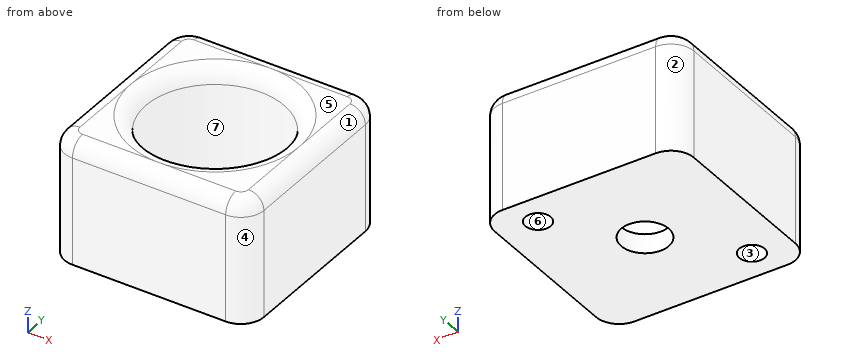
from build123d import *

# Parameters (mm, degrees)
F0_W     = 26
F0_H     = 26
F1_DEPTH = 16
F2_R     = 9
F3_DEPTH = 13.5
F4_R     = 1.65
F4_R_2   = 3.1
F5_DEPTH = 13
F6_R     = 3
F7_R     = 1.99999


# Not quite as in the source:
# - a fillet or chamfer is up to 0.001 mm smaller than in the source, because OpenCascade refuses the exact size


with BuildPart() as f1:
    # F0 (on Top) → F1 (new body)
    with BuildSketch(Plane.XY):
        Rectangle(F0_W, F0_H)
    extrude(amount=F1_DEPTH)

    # F2 (on face) → F3 (cut)
    with BuildSketch(Plane.XY.offset(16)):
        Circle(F2_R)
    extrude(amount=-F3_DEPTH, mode=Mode.SUBTRACT)

    # F4 (on face) → F5 (cut)
    with BuildSketch(Plane(origin=(0, 0, 0), x_dir=(1, 0, 0), z_dir=(0, 0, -1))):
        with Locations((8, -9)):
            Circle(F4_R)
        Circle(F4_R_2)
        with Locations((-8, 9)):
            Circle(F4_R)
    extrude(amount=-F5_DEPTH, mode=Mode.SUBTRACT)

    # F6
    f6_edges = [f1.edges().sort_by_distance(p)[0] for p in [
        (-13, 13, 8),
        (13, 13, 8),
        (-13, -13, 8),
        (13, -13, 8),
    ]]
    fillet(f6_edges, radius=F6_R)

    # F7 (radius 2 in the source; OpenCascade refuses exactly that, so slightly less here)
    f7_edges = [f1.edges().sort_by_distance(p)[0] for p in [
        (-12.12132, -12.12132, 16),
        (-13, 0, 16),
        (-12.12132, 12.12132, 16),
        (0, 13, 16),
        (12.12132, 12.12132, 16),
        (13, 0, 16),
        (12.12132, -12.12132, 16),
        (0, -13, 16),
        (-9, 0, 16),
    ]]
    fillet(f7_edges, radius=F7_R)


solid = f1.part
Here's how the part is built. I have some questions about the finished solid (model axes, mm). Face numbers are marked on the shaded views. A direction names the side the tool comes from. Round coordinates to 2 decimals unless told otherwise and drop trailing zeros. Write each loop counter-clockwise with the first axis right and the second up, starting at its lowest first coordinate (ties: lowest second). Pieces come first, ordered by that corner, then holes.
1. Suppose I cut it at D-D (z = 7.75). List the corners of the cut face in (x, y) for me.
2. Will these pins go through, and if not, where does the flat tip stop? pin 1 Ø1.7 at (x, y) = (8.5, 8.5) entering from -Z; pin 2 Ø1 at (x, y) = (6.5, -4) entering from +Z; pin 3 Ø3.5 at (x, y) = (-7.5, -8.5) entering from -Z; pin 4 Ø5.5 at (x, y) = (0, 0) entering from -Z (3 decimals).
3. I need wall thicknesses on L1, parallel to X at y = 0, z = 1.15; L2, parallel to Y at x = 0, z = 8.25. Which ranges of each line are inside material? Lowest first, please.
4. Suppose I cut it at B-B (z = 1.25). List the corners of the cut face in (x, y) for me, and give its area (3 significant figures).
5. For the marked faces 5, 6 and 7, which set-ups out of +Z, -Z, +X, -X, +Y, -Y let a thin tool reach every point of the face, with its end or its side?
6. If we mould it in two halves opening along Y, with no side actions, what happens to the marked faces 1, 2, 3 and 4? For each: released by +Y, released by -Y, zero draft, split by the parting line, or undercut.
Answer sheet:
1. outline: (-13, -10) arc R3 ccw to (-10, -13) - (10, -13) arc R3 ccw to (13, -10) - (13, 10) arc R3 ccw to (10, 13) - (-10, 13) arc R3 ccw to (-13, 10) - close; hole circle Ø3.3 at (-8, -9); hole circle Ø18 at (0, 0); hole circle Ø3.3 at (8, 9)
2. pin 1: stops at z = 13
2. pin 2: stops at z = 2.5
2. pin 3: stops at z = 0
2. pin 4: passes through
3. L1: x = -13 to -3.1, 3.1 to 13
3. L2: y = -13 to -9, 9 to 13
4. outline: (-13, -10) arc R3 ccw to (-10, -13) - (10, -13) arc R3 ccw to (13, -10) - (13, 10) arc R3 ccw to (10, 13) - (-10, 13) arc R3 ccw to (-13, 10) - close; hole circle Ø3.3 at (-8, -9); hole circle Ø6.2 at (0, 0); hole circle Ø3.3 at (8, 9)
4. area: 621 mm2
5. face 5: +Z, +X, -X, +Y, -Y
5. face 6: -Z
5. face 7: +Z
6. face 1: zero draft
6. face 2: released by +Y
6. face 3: undercut
6. face 4: released by -Y
